Work out the finished part from the listing and answer in its coordinate system (mm). A direction names the side the tool comes from. Give positions to 0.01 mm unless a question says otherwise; leave off trailing zeros. Loops run counter-clockwise (first coordinate to the right, second up) from the corner with the lowest first, then second, coordinate; pieces in that order, holes last. Notation, with made-up numbers: (67, 80.25) - (89, 80.25) arc R11 ccw to (89, 99.25) - close; hole circle Ø10 at (25, -6.75). An arc over 180 degrees is marked (long way). One line per question, with ' | ' between items.
from build123d import *

# Parameters (mm, degrees)
EXTRUDE1_DEPTH        = 30
FILLET1_R             = 5
M5_TAPPED_HOLE1_D     = 4.2
M6_TAPPED_HOLE1_D     = 5
M6_TAPPED_HOLE1_DEPTH = 20
M6_TAPPED_HOLE1_TIP   = 1.502151548


with BuildPart() as part:
    # Sketch1 → Extrude1 (new body)
    with BuildSketch(Plane.XY):
        with BuildLine():
            Line((-25, 32.5), (25, 32.5))
            Line((25, 32.5), (25, -20))
            Line((25, -20), (8.5, -20))
            Line((8.5, -20), (8.5, -11.124297731))
            ThreePointArc((8.5, -11.124297731), (0, 14), (-8.5, -11.124297731))
            Line((-8.5, -11.124297731), (-8.5, -20))
            Line((-8.5, -20), (-25, -20))
            Line((-25, -20), (-25, 32.5))
        make_face()
    extrude(amount=EXTRUDE1_DEPTH)

    # Fillet1
    fillet1_edges = [part.edges().sort_by_distance(p)[0] for p in [
        (-8.5, -20, 15),
        (-25, -20, 15),
        (25, -20, 15),
        (8.5, -20, 15),
        (8.5, -11.124297731, 15),
        (-8.5, -11.124297731, 15),
    ]]
    fillet(fillet1_edges, radius=FILLET1_R)

    # M5 Tapped Hole1 (through all)
    with Locations(Plane(origin=(0, 0, 0), x_dir=(-1, 0, 0), z_dir=(0, 0, -1))):
        with Locations((-13.588507986, 13.279776004), (13.279776004, 13.588507986), (18.998745808, 0.218306478), (13.588507986, -13.279776004), (-13.279776004, -13.588507986), (-18.998745808, -0.218306478)):
            Hole(M5_TAPPED_HOLE1_D / 2)

    # M6 Tapped Hole1
    with Locations(Plane(origin=(0, 32.5, 0), x_dir=(1, 0, 0), z_dir=(0, 1, 0))):
        with Locations((-17.5, -15), (17.5, -15)):
            Hole(M6_TAPPED_HOLE1_D / 2, depth=M6_TAPPED_HOLE1_DEPTH)
            with Locations((0, 0, -(M6_TAPPED_HOLE1_DEPTH + M6_TAPPED_HOLE1_TIP / 2))):  # 118° drill point
                Cone(0, M6_TAPPED_HOLE1_D / 2, M6_TAPPED_HOLE1_TIP, mode=Mode.SUBTRACT)


solid = part.part
1. Determine the mould class of faces 6 (the cylindrical face through (10, -18.57, 15.21)), 7 (the flat face through (0, 32.5, 15)), 8 (the cylindrical face through (-17.06, -0.59, 15.21)) for opening direction Y: +Y half, -Y half, draft (parallel to the pull), parting line (faces both ways), or undercut.
Evaluation:
face 6: -Y half | face 7: +Y half | face 8: undercut
2. Find section B-B on y = 4. Write down the section's boundary in (x, z), then the cut area to 3 significant figures.
Evaluation:
outline: (-25, 0) - (-13.42, 0) - (-13.42, 30) - (-25, 30) - close; (13.42, 0) - (25, 0) - (25, 30) - (13.42, 30) - close | area: 695 mm2
3. Which of the six approach directions +Z, -Z, +X, -X, +Y, -Y give full straight-line access (tool end or side, diameter ignored) to faces 1 (the cylindrical face through (-8.886, -11.442, 15.21)), 2 (the cylindrical face through (-19.81, 22.36, 15.96)), 3 (the flat face through (0, 18, 0)), 4 (the flat face through (-17, -20, 15)), 5 (the flat face through (-8.5, -14, 15))?
Evaluation:
face 1: +Z, -Z | face 2: +Y | face 3: -Z, +X, -X, +Y, -Y | face 4: +Z, -Z, +X, -X, -Y | face 5: +Z, -Z, -Y
4. Flat-ended cylindrical pins translate along their axes: pin 1 (3 mm diameter, centred on x = 1, z = 15.5, fed in from -Y) (3 decimals); pin 2 (3 mm diameter, centred on x = 17.5, z = 15, fed in from +Y); pin 3 (4 mm diameter, centred on x = 5.5, z = 15, fed in from -Y). Find the tip coordinate at first contact, or state that the pin passes through.
Evaluation:
pin 1: y = 13.775 | pin 2: y = 11.9 | pin 3: y = 11.82
5. Find section C-C on z = 10.5. Write down the section's boundary in (x, y), then the cut area to 3 significant figures.
Evaluation:
outline: (-25, -15) arc R5 ccw to (-20, -20) - (-13.5, -20) arc R5 ccw to (-8.5, -15) - (-8.5, -13.37) arc R5 ccw to (-9.95, -9.85) arc R14 cw (long way) to (9.95, -9.85) arc R5 ccw to (8.5, -13.37) - (8.5, -15) arc R5 ccw to (13.5, -20) - (20, -20) arc R5 ccw to (25, -15) - (25, 32.5) - (-25, 32.5) - close; hole circle Ø4.2 at (-19, 0.22); hole circle Ø4.2 at (-13.59, -13.28); hole circle Ø4.2 at (-13.28, 13.59); hole circle Ø4.2 at (13.28, -13.59); hole circle Ø4.2 at (13.59, 13.28); hole circle Ø4.2 at (19, -0.22) | area: 1,790 mm2
6. Consider L1, parallel to X at y = 0, z = 15.25; L2, parallel to X at y = 24, z = 15; L3, parallel to X at y = -0.5, z = 6.5. Determine where each line is inside the solid, lowest interval first.
Evaluation:
L1: -25 to -21.09, -16.91 to -14, 14 to 16.91, 21.09 to 25 | L2: -25 to -20, -15 to 15, 20 to 25 | L3: -25 to -20.97, -17.03 to -13.99, 13.99 to 16.92, 21.08 to 25
7. Find section D-D on x = -2. Write down the section's boundary in (y, z), then the cut area to 3 significant figures.
Evaluation:
outline: (13.86, 0) - (32.5, 0) - (32.5, 30) - (13.86, 30) - close | area: 559 mm2
8. Find section A-A on y = 24.5. Write down the section's boundary in (x, z), then the cut area to 3 significant figures.
Evaluation:
outline: (-25, 0) - (25, 0) - (25, 30) - (-25, 30) - close; hole circle Ø5 at (-17.5, 15); hole circle Ø5 at (17.5, 15) | area: 1,460 mm2
